Part model, mm, in its own coordinate system. A direction names the side the tool comes from. Round coordinates to 2 decimals unless told otherwise and drop trailing zeros. Order: outer loops, then holes, each group sorted by start corner. A loop starts at its lowest first (then second) coordinate and runs counter-clockwise, first axis right, second up. Notation, with made-up numbers: (-21.75, 17.5) -> (34.25, 17.5) arc R21 ccw to (34.25, 42.5) -> close; hole circle Ø5 at (-24.5, -14). An arc over 180 degrees is marked (long way). Answer as a JSON object with one key per item and string values. Group by question number.
Autodesk Inventor part; units mm, degrees
ref_plane "YZ Plane" through (0, 0, 0) normal (1, 0, 0) x (0, 1, 0)
ref_plane "XZ Plane" through (0, 0, 0) normal (0, 1, 0) x (-1, 0, 0)
ref_plane "XY Plane" through (0, 0, 0) normal (0, 0, 1) x (1, 0, 0)
sketch "Sketch1" plane through (0, 0, 0) normal (0, 0, 1) x (1, 0, 0)
  line L0 (-59.9006, 6.3636) -> (-15.4506, 6.3636)
  line L1 (-15.4506, 6.3636) -> (-15.4506, -12.6864)
  line L2 (-15.4506, -12.6864) -> (-59.9006, -12.6864)
  line L3 (-59.9006, -12.6864) -> (-59.9006, 6.3636)
  line L4 (-63.0756, 9.5386) -> (-12.2756, 9.5386)
  line L5 (-12.2756, 9.5386) -> (-12.2756, -15.8614)
  line L6 (-12.2756, -15.8614) -> (-63.0756, -15.8614)
  line L7 (-63.0756, -15.8614) -> (-63.0756, 9.5386)
  point P0 (0, 0)
  dimension "d2" = 3.175
  dimension "d5" = 50.8
  dimension "d6" = 25.4
extrude "Extrusion1" add sketch "Sketch1" along normal blind 457.2
sketch "Sketch4" plane through (-63.0756, 9.5386, 0) normal (0, 1, 0) x (1, 0, 0)
  circle A0 centre (24.9171, -25.4) radius 14.2621
  line L0 (0, 0) -> (50.8, 0)
  point P0 (63.0756, 0)
  dimension "d13" = 28.5242
  dimension "d14" = 25.4
extrude "Extrusion4" cut sketch "Sketch4" against normal through all
sketch "Sketch2" plane through (-63.0756, 9.5386, 0) normal (0, 1, 0) x (1, 0, 0)
  line L0 (1.5875, -157.1625) -> (49.2125, -157.1625)
  line L1 (49.2125, -157.1625) -> (49.2125, -204.7875)
  line L2 (49.2125, -204.7875) -> (1.5875, -204.7875)
  line L3 (1.5875, -204.7875) -> (1.5875, -157.1625)
  line L4 (50.8, -457.2) -> (0, -457.2)
  circle A0 centre (24.9171, -25.4) radius 14.2621
  line L5 (0, 0) -> (50.8, 0)
  point P0 (63.0756, 0)
  point P1 (25.4, -204.7875)
  point P2 (25.4, -457.2)
  dimension "d7" = 47.625
  dimension "d8" = 47.625
  dimension "d24" = 157.1625
extrude "Extrusion2" cut sketch "Sketch2" against normal up to surface (22.225 mm away) contours L0 L1 L2 L3
sketch "Sketch9" plane through (-59.9006, -12.6864, 0) normal (0, 1, 0) x (1, 0, 0)
  circle A0 centre (21.7421, -180.975) radius 16.7645
  line L0 (-1.5875, -204.7875) -> (-1.5875, -157.1625)
  circle A1 centre (21.7421, -25.4) radius 14.2621
  circle A2 centre (3.4541, -199.263) radius 1.7
  circle A3 centre (40.0301, -199.263) radius 1.7
  circle A4 centre (40.0301, -162.687) radius 1.7
  circle A5 centre (3.4541, -162.687) radius 1.7
  point P0 (59.9006, 0)
  point P1 (-1.5875, -180.975)
  dimension "d34" = 18.288
  dimension "d35" = 18.288
  dimension "d38" = 360
extrude "Extrusion8" cut sketch "Sketch9" against normal through all contours A0 | A2 | A3 | A4 | A5
sketch "Sketch10" plane through (-63.0756, 9.5386, 0) normal (0, 1, 0) x (1, 0, 0)
  circle A0 centre (25.4, -349.25) radius 14.2875
  line L0 (50.8, -457.2) -> (0, -457.2)
  line L1 (0, 0) -> (50.8, 0)
  point P0 (63.0756, 0)
  point P1 (25.4, -457.2)
  dimension "d42" = 28.575
  dimension "d43" = 349.25
extrude "Extrusion9" cut sketch "Sketch10" against normal through all
equation "\"d8\" = d7"
equation "\"d35\" = d34"
properties part number "1x2 arm"
Q1. Band-saw the part on B-B (y = 2.5). List the corners of the cut face in (x, z), plus the area to 3 significant figures.
Q2. Two-plate mould, pull along Y, no slides. Class faces 4 (the flat face through (-37, -15.861, 225)), 5 (the flat face through (-59.901, -3, 329)), 6 (the cylindrical face through (-40.77, -14.25, 363.2)): +Y half, -Y half, draft (parallel to the pull), parting line (faces both ways), or undercut.
Q3. Drop a flat-ended pin along its axis: pin 1 Ø3 at (x, y) = (-30, 3) entering from -Z. Give the stop position or say it passes through.
Q4. Band-saw the part on A-A (z = 25.4). List the corners of the cut face in (x, y).
Q5. Band-saw the part on D-D (x = -30.5). Count the separate pieces of the cut face and the enclosed holes in it, plus the area to 3 significant figures.
Q6. Band-saw the part on C-C (z = 295). List the corners of the cut face in (x, y).
Q7. Wall check: line 1 (Z direction, x = -15, y = -9.5); line 2 (X direction, y = 8.5, z = 349.25); line 3 (Y direction, x = -50, z = 330.5). Give the ranges that are in metal, low to high. Write a range as [from, to].
Q8. Which spindle directions (+Z, -Z, +X, -X, +Y, -Y) get a long thin tool onto all of the face, cutting with end or side? Do faces 1 (the cylindrical face through (-40.341, -14.252, 164.353)), 2 (the flat face through (-38, 7, 157.162)), 3 (the flat face through (-38, 6.364, 77)). Say none if no direction does.
Completed:
{
 "1": {"outline": "(-63.08, 0) -> (-59.9, 0) -> (-59.9, 157.16) -> (-61.49, 157.16) -> (-61.49, 204.79) -> (-59.9, 204.79) -> (-59.9, 457.2) -> (-63.08, 457.2) -> close; (-15.45, 0) -> (-12.28, 0) -> (-12.28, 457.2) -> (-15.45, 457.2) -> (-15.45, 204.79) -> (-13.86, 204.79) -> (-13.86, 157.16) -> (-15.45, 157.16) -> close", "area": "2,750 mm2"},
 "2": {"face 4": "-Y half", "face 5": "undercut", "face 6": "draft"},
 "3": {"pin 1": "through"},
 "4": {"outline": "(-63.08, -15.86) -> (-52.42, -15.86) -> (-52.42, -12.69) -> (-59.9, -12.69) -> (-59.9, 6.36) -> (-52.42, 6.36) -> (-52.42, 9.54) -> (-63.08, 9.54) -> close; (-23.9, -15.86) -> (-12.28, -15.86) -> (-12.28, 9.54) -> (-23.9, 9.54) -> (-23.9, 6.36) -> (-15.45, 6.36) -> (-15.45, -12.69) -> (-23.9, -12.69) -> close"},
 "5": {"separate pieces": "8", "enclosed holes": "0", "area": "2,350 mm2"},
 "6": {"outline": "(-63.08, -15.86) -> (-12.28, -15.86) -> (-12.28, 9.54) -> (-63.08, 9.54) -> close; hole (-59.9, -12.69) -> (-15.45, -12.69) -> (-15.45, 6.36) -> (-59.9, 6.36) -> close"},
 "7": {"line 1": "[0, 157.16], [204.79, 457.2]", "line 2": "[-63.08, -51.96], [-23.39, -12.28]", "line 3": "[-15.86, -12.69], [6.36, 9.54]"},
 "8": {"face 1": "+Y, -Y", "face 2": "+Y", "face 3": "+Z, -Z"}
}
